The listing builds one solid part. Answer for the finished solid, in the listing's coordinates (mm). A direction names the side the tool comes from. Round coordinates to 2 decimals unless told otherwise and drop trailing zeros. Write each loop counter-clockwise with the first axis right and the second up, starting at its lowest first coordinate (ties: lowest second). Pieces come first, ordered by that corner, then holes. Notation, with made-up numbers: M 19,-13 L 27,-13 A30 ccw 27,21 Z; hole C 77,47 d5. An arc over 180 degrees is marked long. Write each question's results on one line, items separated by ' | '.
from build123d import *

# Parameters (mm, degrees)
BOSS_EXTRUDE1_DEPTH   = 20
BOSS_EXTRUDE1_2_DEPTH = 20
BOSS_EXTRUDE1_3_DEPTH = 20
BOSS_EXTRUDE1_4_DEPTH = 20
SKETCH2_W             = 20
SKETCH2_H             = 20
BOSS_EXTRUDE2_DEPTH   = 20
CUT_EXTRUDE1_DEPTH    = 31
BOSS_EXTRUDE3_DEPTH   = 30
SKETCH5_R             = 2.7
CUT_EXTRUDE2_DEPTH    = 30
SKETCH6_R             = 5
CUT_EXTRUDE3_DEPTH    = 30
FILLET1_R             = 7
FILLET3_R             = 1
FILLET4_R             = 0.75


# Some blends are built 0.0001 mm under size
with BuildPart() as part:
    # Sketch1 → Boss-Extrude1 (new body)
    with BuildSketch(Plane(origin=(0, 0, 0), x_dir=(1, 0, 0), z_dir=(0, 1, 0))):
        Polygon((-10, -2.8), (-10, 2.8), (-7.7, 2.8), (-7.7, 5.58), (-7.135634919, 5.58), (-4.28, 2.724365081), (-4.28, -2.724365081), (-7.135634919, -5.58), (-7.7, -5.58), (-7.7, -2.8), align=None)
    extrude(amount=BOSS_EXTRUDE1_DEPTH)



with BuildPart() as body_2:
    # Sketch1 → Boss-Extrude1 2 (new body)
    with BuildSketch(Plane(origin=(0, 0, 0), x_dir=(1, 0, 0), z_dir=(0, 1, 0))):
        Polygon((10, 2.8), (7.7, 2.8), (7.7, 5.58), (7.135634919, 5.58), (4.28, 2.724365081), (4.28, -2.724365081), (7.135634919, -5.58), (7.7, -5.58), (7.7, -2.8), (10, -2.8), align=None)
    extrude(amount=BOSS_EXTRUDE1_2_DEPTH)


with BuildPart() as body_3:
    # Sketch1 → Boss-Extrude1 3 (new body)
    with BuildSketch(Plane(origin=(0, 0, 0), x_dir=(1, 0, 0), z_dir=(0, 1, 0))):
        Polygon((2.8, -10), (-2.8, -10), (-2.8, -7.7), (-5.58, -7.7), (-5.58, -7.135634919), (-2.724365081, -4.28), (2.724365081, -4.28), (5.58, -7.135634919), (5.58, -7.7), (2.8, -7.7), align=None)
    extrude(amount=BOSS_EXTRUDE1_3_DEPTH)


with BuildPart() as body_4:
    # Sketch1 → Boss-Extrude1 4 (new body)
    with BuildSketch(Plane(origin=(0, 0, 0), x_dir=(1, 0, 0), z_dir=(0, 1, 0))):
        Polygon((-2.8, 10), (-2.8, 7.7), (-5.58, 7.7), (-5.58, 7.135634919), (-2.724365081, 4.28), (2.724365081, 4.28), (5.58, 7.135634919), (5.58, 7.7), (2.8, 7.7), (2.8, 10), align=None)
    extrude(amount=BOSS_EXTRUDE1_4_DEPTH)


with BuildPart() as part_1:
    add(part.part)

    add(body_2.part)  # Boss-Extrude2 merges body 2

    add(body_3.part)  # Boss-Extrude2 merges body 3

    add(body_4.part)  # Boss-Extrude2 merges body 4
    # Sketch2 → Boss-Extrude2 (add)
    with BuildSketch(Plane.XZ):
        Rectangle(SKETCH2_W, SKETCH2_H)
    extrude(amount=BOSS_EXTRUDE2_DEPTH)

    # Sketch3 → Cut-Extrude1 (cut, through all)
    with BuildSketch(Plane(origin=(10, 0, 0), x_dir=(0, 0, -1), z_dir=(1, 0, 0))):
        Polygon((10.596673941, -8.137212268), (10.596673941, -38.345549702), (-10.411138478, -38.345549702), (-10.411138478, -2.402671747), align=None)
    extrude(amount=-CUT_EXTRUDE1_DEPTH, mode=Mode.SUBTRACT)

    # Sketch4 → Boss-Extrude3 (add)
    with BuildSketch(Plane(origin=(10, 0, 0), x_dir=(0, 0, -1), z_dir=(1, 0, 0))):
        Polygon((10, -7.974337104), (10, 0), (-10, 0), (-10, -2.51490096), align=None)
    extrude(amount=BOSS_EXTRUDE3_DEPTH)

    # Sketch5 → Cut-Extrude2 (cut)
    with BuildSketch(Plane(origin=(0, 0, 0), x_dir=(1, 0, 0), z_dir=(0, 1, 0))):
        with Locations(Location((28.5, 0, 0), (0, 0, 270))):
            Circle(SKETCH5_R)
    extrude(amount=-CUT_EXTRUDE2_DEPTH, mode=Mode.SUBTRACT)

    # Sketch6 → Cut-Extrude3 (cut)
    with BuildSketch(Plane(origin=(0, -1.5, 0), x_dir=(1, 0, 0), z_dir=(0, 1, 0))):
        with Locations(Location((28.5, 0, 0), (0, 0, 270))):
            Circle(SKETCH6_R)
    extrude(amount=-CUT_EXTRUDE3_DEPTH, mode=Mode.SUBTRACT)

    # Fillet1
    # the kernel refuses this fillet: 7 mm, written as the material it takes off along each edge
    with BuildSketch(Plane(origin=(-10, -12.582734088, -26.882318479), x_dir=(0, 0.9647039130954433, -0.26333697054978655), z_dir=(0, 0.26333697054978655, 0.9647039130954435))) as fillet1_piece_1:
        with BuildLine():
            CenterArc((FILLET1_R, -FILLET1_R), FILLET1_R, 90, 90)
            Line((0, -FILLET1_R), (0, 0))
            Line((0, 0), (FILLET1_R, 0))
        make_face()
    extrude(amount=55.731749637, mode=Mode.SUBTRACT)

    # Fillet3
    fillet3_edges = [part_1.edges().sort_by_distance(p)[0] for p in [
        (4.152182541, 0, -5.707817459),
        (5.58, 0, -7.417817459),
        (4.19, 0, -7.7),
        (2.8, 0, -8.85),
        (-2.8, 0, -8.85),
        (-4.19, 0, -7.7),
        (-5.58, 0, -7.417817459),
        (-4.152182541, 0, -5.707817459),
        (0, 0, -4.28),
        (4.28, 0, 0),
        (5.707817459, 0, -4.152182541),
        (7.417817459, 0, -5.58),
        (7.7, 0, -4.19),
        (8.85, 0, -2.8),
        (10, 0, 0),
        (8.85, 0, 2.8),
        (7.7, 0, 4.19),
        (5.707817459, 0, 4.152182541),
        (7.417817459, 0, 5.58),
        (2.8, 0, 8.85),
        (4.19, 0, 7.7),
        (5.58, 0, 7.417817459),
        (4.152182541, 0, 5.707817459),
        (0, 0, 4.28),
        (-4.152182541, 0, 5.707817459),
        (-5.58, 0, 7.417817459),
        (-2.8, 0, 8.85),
        (-4.19, 0, 7.7),
        (-8.583774042, 0, 2.8),
        (-7.7, 0, 4.19),
        (-7.417817459, 0, 5.58),
        (-5.707817459, 0, 4.152182541),
        (-4.28, 0, 0),
        (-5.707817459, 0, -4.152182541),
        (-7.417817459, 0, -5.58),
        (-7.7, 0, -4.19),
        (-8.79791333, 0, -2.8),
    ]]
    fillet(fillet3_edges, radius=FILLET3_R)

    # Fillet4
    fillet4_edges = [part_1.edges().sort_by_distance(p)[0] for p in [
        (28.5, 0, -2.7),
        (28.5, -6.609478068, -5),
        (28.5, -1.5, -5),
        (28.5, -1.5, -2.7),
    ]]
    fillet(fillet4_edges, radius=FILLET4_R - 0.0001)  # a hair under: the kernel refuses the full size


solid = part_1.part
1) A tool of negligible diameter and unlimited length cuts with its end or side. For faces 1 (the face through (-4, 10, -7.7)), 2 (the face through (2.8, 10, -9)), 3 (the face through (-9, 10, 2.8)), from which of +Z, -Z, +X, -X, +Y, -Y can it reach the whole face along a straight path? Write none if from no direction.
Return value:
face 1: -Z, -X, +Y | face 2: -Z, +X, +Y | face 3: +Z, -X, +Y
2) Each of these flat-tipped pins is pushed along its axis until it touches: pin 1 (1.2 mm diameter, centred on y = 7.5, z = -9, fed in from +X); pin 2 (2.5 mm diameter, centred on x = 9, y = 7, fed in from -Z); pin 3 (2.5 mm diameter, centred on y = 14, z = -9, fed in from -X); pin 4 (3 mm diameter, centred on y = 3, z = 3, fed in from -X). Where does it stop, or does it pass through?
Return value:
pin 1: x = 2.8 | pin 2: z = -2.8 | pin 3: x = -2.8 | pin 4: x = -10
3) Section B-B (y = 17) is taken. State how many separate pieces and enclosed holes the cut face has, then the cut area to 3 significant figures.
Return value:
separate pieces: 4 | enclosed holes: 0 | area: 172 mm²
4) Find the intervals of material crossed by line 1 (X direction, y = 5, z = 4.5); line 2 (Z direction, x = 5, y = 14.5); line 3 (Y direction, x = 22.5, z = 5.25), in increasing order.
Return value:
line 1: -7.7 to -6.06, -2.94 to 2.94, 6.06 to 7.7 | line 2: -7.7 to -6.56, -3.44 to 3.44, 6.56 to 7.7 | line 3: -3.81 to 0
5) The mould has two halves that part along X. Classify faces 4 (the face through (-7.7, 10, 4)), 5 (the face through (4, 10, -7.7)), 6 (the face through (-4.341, 0.285, -5.471)), 7 (the face through (3.101, 0.285, 9.122)): +X half, -X half, draft (parallel to the pull), parting line (faces both ways), or undercut.
Return value:
face 4: -X half | face 5: draft | face 6: undercut | face 7: +X half
6) Section A-A (x = 1.5) is taken. Determine the outline of the cut face in (y, z), then the cut area to 3 significant figures.
Return value:
outline: M -7.97,-10 L 20,-10 L 20,-4.28 L 1,-4.28 A1 cw 0,-3.28 L 0,3.28 A1 cw 1,4.28 L 20,4.28 L 20,10 L -2.51,10 Z | area: 334 mm²
7) Section C-C (x = 17) is taken. Determine the outline of the cut face in (y, z).
Return value:
outline: M -7.97,-10 L 0,-10 L 0,10 L -2.51,10 Z
